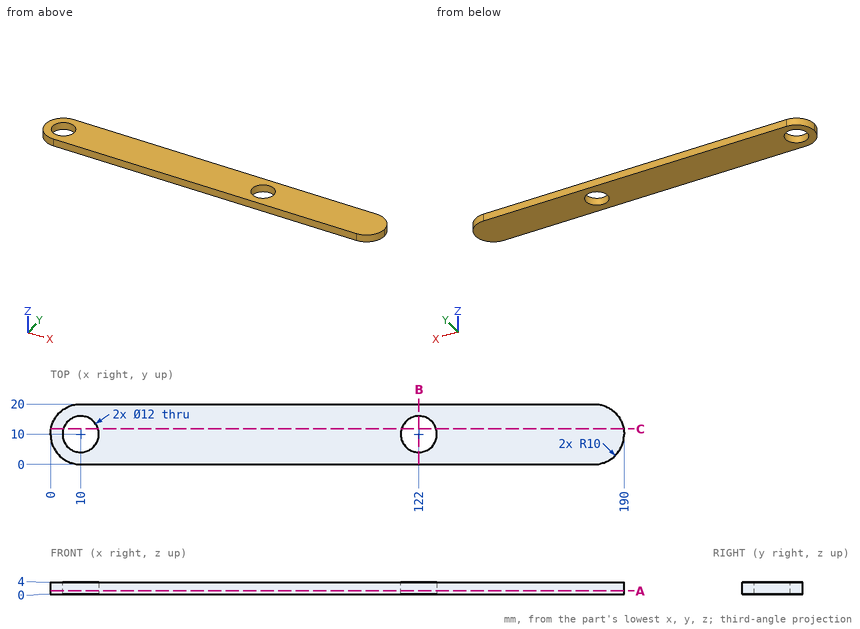
Can you work these out from the drawing? Everything is in mm from the part's minimum corner. Coordinates: 2 decimals unless noted, no trailing zeros. Order: outer loops, then holes, each group sorted by start corner. A loop starts at its lowest first (then second) coordinate and runs counter-clockwise, first axis right, second up. Notation, with made-up numbers: M -19.5,34.25 L 27.5,34.25 A32 cw 27.5,66.25 Z; hole C 39,15 d2. An arc over 180 degrees is marked long. Answer as CSV lines item,"result". Start each with the question number.
1. I want a section at A-A, the plane z = 1.2. Count the separate pieces of the cut face and the enclosed holes in it, and give its area (3 significant figures).
2. I want a section at C-C, the plane y = 11.75. Write out the boundary of the cut face in (x, z).
3. I need wall thicknesses on line 1 (Y direction, x = 122, z = 2.8); line 2 (X direction, y = 7.5, z = 1.3); line 3 (X direction, y = 8.5, z = 0.6). Which ranges of each line are inside material? Lowest first, please. Write a range as [from, to].
4. I want a section at B-B, the plane x = 122. Write out the boundary of the cut face in (y, z).
5. For pin 1 (2 mm diameter, centred on y = 4.5, z = 2, fed in from +X); pin 2 (2 mm diameter, centred on y = 9, z = 1, fed in from +X); pin 3 (7 mm diameter, centred on x = 122, y = 10, fed in from -Z), each with a flat end and sliding along its axis, tell me the tip position at first contact or that it passes through.
Recorded:
1,separate pieces,"1"
1,enclosed holes,"2"
1,area,"3,490 mm2"
2,outline,"M 0.15,0 L 4.26,0 L 4.26,4 L 0.15,4 Z; M 15.74,0 L 116.26,0 L 116.26,4 L 15.74,4 Z; M 127.74,0 L 189.85,0 L 189.85,4 L 127.74,4 Z"
3,line 1,"y = [0, 4], [16, 20]"
3,line 2,"x = [0.32, 4.55], [15.45, 116.55], [127.45, 189.68]"
3,line 3,"x = [0.11, 4.19], [15.81, 116.19], [127.81, 189.89]"
4,outline,"M 0,0 L 4,0 L 4,4 L 0,4 Z; M 16,0 L 20,0 L 20,4 L 16,4 Z"
5,pin 1,"stops at x = 188.93"
5,pin 2,"stops at x = 190"
5,pin 3,"passes through"
